The drawing under review shows one solid part. Ordinate dimensions are in mm from its lowest x, y, z. A direction names the side the tool comes from. Give positions to 0.01 mm unless a question says otherwise; leave off trailing zeros. Write each loop counter-clockwise with the first axis right and the second up, starting at its lowest first coordinate (ties: lowest second). Pieces come first, ordered by that corner, then holes. Notation, with made-up numbers: (40.25, -14) -> (70.25, -14) arc R15 cw to (70.25, 5) -> close; hole circle Ø5 at (-36.5, -14.5). An arc over 180 degrees is marked (long way). Answer as a JSON object with one key per item and string values.
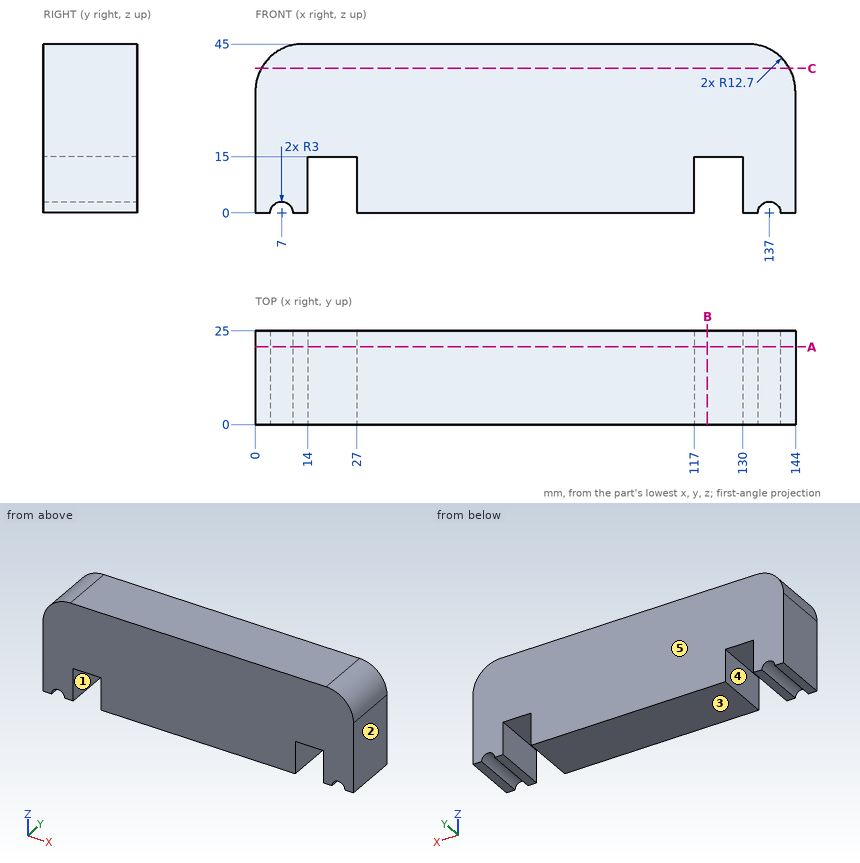
(1) We need section B-B, the plane x = 120.5. State the section outline as (y, z) points.
Here are the results:
{"outline": "(0, 15) -> (25, 15) -> (25, 45) -> (0, 45) -> close"}
(2) Clearance check with flat-ended pins moving along their axes: pin 1 (14.5 mm diameter, centred on x = 120.5, y = 10.5, fed in from -Z); pin 2 (4 mm diameter, centred on x = 22, y = 16, fed in from -Z). State where each tip first meets the part, or that it passes through.
Here are the results:
{"pin 1": "stops at z = 0", "pin 2": "stops at z = 15"}
(3) We need section C-C, the plane z = 38.5. State the section outline as (x, y) points.
Here are the results:
{"outline": "(1.62, 0) -> (142.38, 0) -> (142.38, 25) -> (1.62, 25) -> close"}
(4) We need section A-A, the plane y = 20.75. State the section outline as (x, z) points, then the cut area to 3 significant figures.
Here are the results:
{"outline": "(0, 0) -> (4, 0) arc R3 cw to (10, 0) -> (14, 0) -> (14, 15) -> (27, 15) -> (27, 0) -> (117, 0) -> (117, 15) -> (130, 15) -> (130, 0) -> (134, 0) arc R3 cw to (140, 0) -> (144, 0) -> (144, 32.3) arc R12.7 ccw to (131.3, 45) -> (12.7, 45) arc R12.7 ccw to (0, 32.3) -> close", "area": "5,990 mm²"}
(5) For the marked faces 4 and 5, list the 3-axis set-ups (+Z, -Z, +X, -X, +Y, -Y) from which the entire face can be reached by the end or side of a thin tool; tool diameter is ignored.
Here are the results:
{"face 4": "-Z, +Y, -Y", "face 5": "+Z, -Z, +X, -X, +Y"}
(6) The part is to be moulded in two halves that separate along X. For the marked faces 1, 2 and 3, say which applies: +X half, -X half, draft (parallel to the pull), parting line (faces both ways), or undercut.
Here are the results:
{"face 1": "undercut", "face 2": "+X half", "face 3": "draft"}
(7) For line 1 along X through (y, z) = (18, 12); line 2 along Z through (x, y) = (127.5, 14.75); line 3 along X through (y, z) = (21.75, 39), list the stretches that pass through material, from the lowest coordinate up.
Here are the results:
{"line 1": "x = 0 to 14, 27 to 117, 130 to 144", "line 2": "z = 15 to 45", "line 3": "x = 1.91 to 142.09"}
